Check sheet for the modelled part. Datum: model origin and axes. Units: mm. A direction names the side the tool comes from. Give positions to 0.01 mm unless a question says otherwise; leave off trailing zeros. Order: outer loops, then holes, each group sorted by start corner. A loop starts at its lowest first (then second) coordinate and runs counter-clockwise, first axis right, second up.
```python
from build123d import *

# Parameters (mm, degrees)
EXTRUDE_1_DEPTH     = 10
SKETCH_3_R          = 1.25
CUT_EXTRUDE_2_DEPTH = 4


with BuildPart() as part:
    # Эскиз1 → Бобышка-Вытянуть1 (new body)
    with BuildSketch(Plane(origin=(0, 0, 0), x_dir=(1, 0, 0), z_dir=(0, 1, 0))):
        Polygon((-13.5, 2), (13.5, 2), (13.5, -6), (20.5, -6), (20.5, -10), (12.2, -10), (12.2, 0), (-12.2, 0), (-12.2, -10), (-20.5, -10), (-20.5, -6), (-13.5, -6), align=None)
    extrude(amount=EXTRUDE_1_DEPTH)

    # Эскиз3 → Вырез-Вытянуть2 (cut)
    with BuildSketch(Plane(origin=(0, 0, 6), x_dir=(-1, 0, 0), z_dir=(0, 0, -1))):
        with Locations((17, 5)):
            Circle(SKETCH_3_R)
    cut_extrude_2 = extrude(amount=-CUT_EXTRUDE_2_DEPTH, mode=Mode.SUBTRACT)

    # Зеркальное отражение1: Вырез-Вытянуть2 across plane
    add(cut_extrude_2.mirror(Plane.ZY), mode=Mode.SUBTRACT)


solid = part.part
```
(1) Cross-section at B-B on x = -17. Enter the section's corners in (y, z).
Response values:
outline: (0, 6) - (3.75, 6) - (3.75, 10) - (0, 10) - close; (6.25, 6) - (10, 6) - (10, 10) - (6.25, 10) - close
(2) Cross-section at C-C on z = 3.5. Enter the section's corners in (x, y).
Response values:
outline: (-13.5, 0) - (-12.2, 0) - (-12.2, 10) - (-13.5, 10) - close; (12.2, 0) - (13.5, 0) - (13.5, 10) - (12.2, 10) - close
(3) Material ranges on L1, parallel to Y at x = -17, z = 8.85; L2, parallel to X at y = 7, z = 6.75; L3, parallel to X at y = 3, z = 4, recorded low to high.
Response values:
L1: y = 0 to 3.75, 6.25 to 10
L2: x = -20.5 to -12.2, 12.2 to 20.5
L3: x = -13.5 to -12.2, 12.2 to 13.5
(4) Gauge pin test, flat ends, axial feed: pin 1 Ø4 at (y, z) = (3, 2.5) entering from -X; pin 2 Ø1.5 at (x, y) = (-17, 5) entering from +Z; pin 3 Ø2 at (x, y) = (-17.5, 3.5) entering from -Z. Record the tip position at first contact, or that the pin passes through.
Response values:
pin 1: stops at x = -13.5
pin 2: passes through
pin 3: stops at z = 6
(5) Release check for a two-part mould opening along Y. For faces 1 (the face through (1.6, 0, -0.5)), 2 (the face through (16.73, 3.78, 7.97)), 3 (the face through (0, 5, -2)) record: released by +Y, released by -Y, zero draft, split by the parting line, or undercut.
Response values:
face 1: released by -Y
face 2: undercut
face 3: zero draft
(6) Set-up check for faces 4 (the face through (13.5, 5, 2)), 5 (the face through (12.2, 5, 5)), 6 (the face through (1.6, 10, -0.5)), 7 (the face through (-20.5, 5, 8)), 8 (the face through (-13.5, 5, 2)): record each of +Z, -Z, +X, -X, +Y, -Y from which the full face is reachable in a straight line by a thin tool's end or side.
Response values:
face 4: -Z, +X, +Y, -Y
face 5: +Z, +Y, -Y
face 6: +Z, -Z, +X, -X, +Y
face 7: +Z, -Z, -X, +Y, -Y
face 8: -Z, -X, +Y, -Y
(7) Cross-section at A-A on z = 8. Enter the section's corners in (x, y).
Response values:
outline: (-20.5, 0) - (-12.2, 0) - (-12.2, 10) - (-20.5, 10) - close; (12.2, 0) - (20.5, 0) - (20.5, 10) - (12.2, 10) - close; hole circle Ø2.5 at (-17, 5); hole circle Ø2.5 at (17, 5)
(8) Cross-section at D-D on y = 7. Enter the section's corners in (x, z).
Response values:
outline: (-20.5, 6) - (-13.5, 6) - (-13.5, -2) - (13.5, -2) - (13.5, 6) - (20.5, 6) - (20.5, 10) - (12.2, 10) - (12.2, 0) - (-12.2, 0) - (-12.2, 10) - (-20.5, 10) - close
